Read the model definition and answer for the solid it produces. Units are mm, in the model's axes. Face numbers are marked on the shaded views. A direction names the side the tool comes from. Round coordinates to 2 decimals unless told otherwise and drop trailing zeros. Write each loop counter-clockwise with the first axis right and the second up, starting at its lowest first coordinate (ties: lowest second). Pieces come first, ordered by that corner, then holes. Notation, with made-up numbers: (-38, 68) - (-10, 68) arc R22 ccw to (-10, 90) - close; hole circle Ø11 at (-32.75, 39). An arc over 180 degrees is marked (long way). Use one line per item in the form item = value. Start each with the question number.
1) The part is cut by section D-D, the plane x = 69.5. Give the vertices of the cut face in (y, z).
2) For the marked faces 1, 2 and 3, determine the directions among +Z, -Z, +X, -X, +Y, -Y from which every point of the face is accessible in a straight line to the end or side of a thin tool.
3) The part is cut by section C-C, the plane z = 114.5. Give the vertices of the cut face in (x, y).
4) Consider line 1 along X through (y, z) = (-7.5, 107); line 2 along Z through (x, y) = (241, -16.5); line 3 along Z through (x, y) = (133, -19.5). Determine where each line is inside the solid, lowest interval first. Write a range as from..to.
5) Each of these flat-tipped pins is pushed along its axis until it touches: pin 1 (1 mm diameter, centred on y = -0.5, z = 3, fed in from +X); pin 2 (11 mm diameter, centred on x = 177.5, y = -13, fed in from -Z); pin 3 (11 mm diameter, centred on x = 262.5, y = -13.5, fed in from +Z). Where does it stop, or does it pass through?
6) The part is cut by section A-A, the plane y = -9. Give the vertices of the cut face in (x, z), plus the area to 3 significant figures.
7) The part is cut by section B-B, the plane x = 34.5. Give the vertices of the cut face in (y, z).
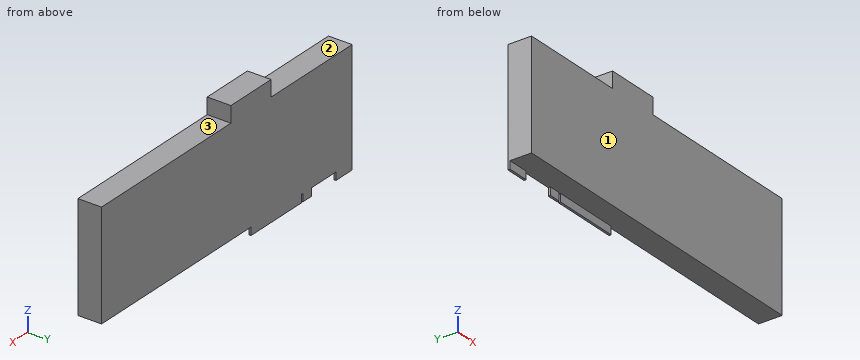
from build123d import *

# Parameters (mm, degrees)
F1_DEPTH = 2
F2_W     = 312
F2_H     = 99.44
F3_DEPTH = 20
F4_W     = 50
F4_H     = 15
F5_DEPTH = 22


with BuildPart() as f1:
    # F0 (on Front) → F1 (new body)
    with BuildSketch(Plane.XZ):
        Polygon((0, 106.68), (0, 0), (20.08, 0), (20.08, 7.24), (50.296851, 7.24), (50.296851, 0), (61.29, 0), (61.29, 7.24), (63.144, 7.24), (63.144, 0), (125.914, 0), (125.914, 7.24), (312, 7.24), (312, 106.68), align=None)
    extrude(amount=F1_DEPTH)

    # F2 (on face) → F3 (join)
    with BuildSketch(Plane.XZ.offset(2)):
        with Locations((156, 56.96)):
            Rectangle(F2_W, F2_H)
    extrude(amount=F3_DEPTH)

    # F4 (on face) → F5 (join)
    with BuildSketch(Plane(origin=(0, 0, 0), x_dir=(-1, 0, 0), z_dir=(0, 1, 0))):
        with Locations((-125.914, 114.18)):
            Rectangle(F4_W, F4_H)
    extrude(amount=-F5_DEPTH)


solid = f1.part
Geometry results:
q1.outline = (-22, 7.24) - (-2, 7.24) - (-2, 0) - (0, 0) - (0, 106.68) - (-22, 106.68) - close
q2.face_1 = +Z, -Z, +X, -X, -Y
q2.face_2 = +Z, -X, +Y, -Y
q2.face_3 = +Z, +X, +Y, -Y
q3.outline = (100.91, -22) - (150.91, -22) - (150.91, 0) - (100.91, 0) - close
q4.line_1 = 100.91..150.91
q4.line_2 = 7.24..106.68
q4.line_3 = 7.24..121.68
q5.pin_1 = 125.91
q5.pin_2 = 7.24
q5.pin_3 = 106.68
q6.outline = (0, 7.24) - (312, 7.24) - (312, 106.68) - (150.91, 106.68) - (150.91, 121.68) - (100.91, 121.68) - (100.91, 106.68) - (0, 106.68) - close
q6.area = 31,800 mm2
q7.outline = (-22, 7.24) - (0, 7.24) - (0, 106.68) - (-22, 106.68) - close
